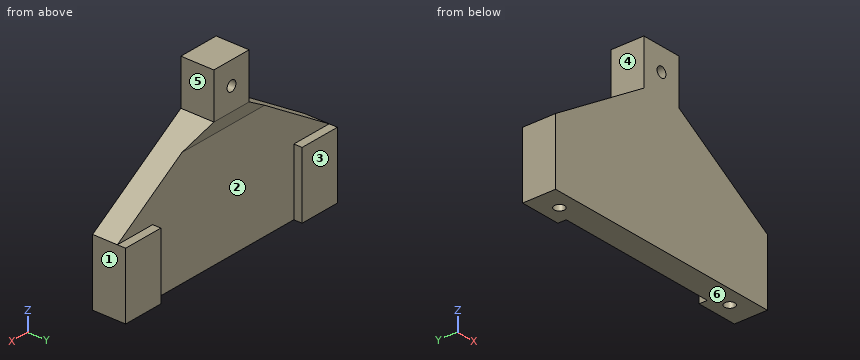
```python
from build123d import *

# Parameters (mm, degrees)
ESQUISSE1_W             = 60
ESQUISSE1_H             = 8
BOSS_EXTRU_1_DEPTH      = 60
ESQUISSE2_R             = 1.25
ENL_V_MAT_EXTRU_1_DEPTH = 15
ESQUISSE3_R             = 1.25
ENL_V_MAT_EXTRU_2_DEPTH = 15
ESQUISSE4_W             = 10
ESQUISSE4_H             = 11
ENL_V_MAT_EXTRU_3_DEPTH = 2
ENL_V_MAT_EXTRU_4_DEPTH = 52
CHANFREIN1_SIZE2        = 4.289013841
CHANFREIN1_SIZE         = 2


with BuildPart() as part:
    # Esquisse1 → Boss.-Extru.1 (new body)
    with BuildSketch(Plane.XY):
        with Locations((30, 4)):
            Rectangle(ESQUISSE1_W, ESQUISSE1_H)
    extrude(amount=BOSS_EXTRU_1_DEPTH)

    # Esquisse2 → Enlèv. mat.-Extru.1 (cut)
    with BuildSketch(Plane(origin=(0, 0, 0), x_dir=(-1, 0, 0), z_dir=(0, 0, -1))):
        with Locations((-54, 4)):
            Circle(ESQUISSE2_R)
        with Locations((-5.75, 4)):
            Circle(ESQUISSE2_R)
    extrude(amount=-ENL_V_MAT_EXTRU_1_DEPTH, mode=Mode.SUBTRACT)

    # Esquisse3 → Enlèv. mat.-Extru.2 (cut)
    with BuildSketch(Plane(origin=(0, 8, 0), x_dir=(1, 0, 0), z_dir=(0, 1, 0))):
        with Locations(Location((30, -37.5, 0), (0, 0, 270))):
            Circle(ESQUISSE3_R)
    extrude(amount=-ENL_V_MAT_EXTRU_2_DEPTH, mode=Mode.SUBTRACT)

    # Esquisse4 → Enlèv. mat.-Extru.3 (cut)
    with BuildSketch(Plane(origin=(0, 8, 0), x_dir=(1, 0, 0), z_dir=(0, 1, 0))):
        Polygon((0, -16), (10, -16), (10, 0), (50, 0), (50, -16), (60, -16), (60, -60), (0, -60), align=None)
        with Locations((30, -37.5)):
            Rectangle(ESQUISSE4_W, ESQUISSE4_H, mode=Mode.SUBTRACT)
    extrude(amount=-ENL_V_MAT_EXTRU_3_DEPTH, mode=Mode.SUBTRACT)

    # Esquisse5 → Enlèv. mat.-Extru.4 (cut)
    with BuildSketch(Plane(origin=(0, 6, 0), x_dir=(1, 0, 0), z_dir=(0, 1, 0))):
        Polygon((60, -16), (35, -32), (35, -43), (25, -43), (25, -32), (0, -16), (-21.594855386, -85.475485762), (75.414479662, -69.930764824), align=None)
    extrude(amount=-ENL_V_MAT_EXTRU_4_DEPTH, mode=Mode.SUBTRACT)

    # Chanfrein1
    chanfrein1_edges = [part.edges().sort_by_distance(p)[0] for p in [
        (30, 6, 32),
    ]]
    chanfrein1_side = [part.faces().sort_by_distance(p)[0] for p in [
        (30, 6.04, 32),
    ]]
    chamfer(chanfrein1_edges, length=CHANFREIN1_SIZE - 0.0001, length2=CHANFREIN1_SIZE2 - 0.0001, reference=chanfrein1_side[0])  # a hair under: the kernel refuses the full size


solid = part.part
```
Could you check a few things on this model? Use its own coordinates, in mm. Face numbers are marked on the shaded views. A direction names the side the tool comes from. Coordinates: 2 decimals unless noted, no trailing zeros. Write each loop counter-clockwise with the first axis right and the second up, starting at its lowest first coordinate (ties: lowest second). Pieces come first, ordered by that corner, then holes. Notation, with made-up numbers: (23, 59.5) -> (77, 59.5) arc R20 ccw to (77, 73.5) -> close; hole circle Ø4 at (78, 21.5). An arc over 180 degrees is marked (long way). Return JSON: item names as keys, results as strings.
(1) I need wall thicknesses on L1, parallel to Y at x = 54, z = 11; L2, parallel to X at y = 2.5, z = 39; L3, parallel to Y at x = 30, z = 9. Which ranges of each line are inside material? Lowest first, please.
Numbers:
{"L1": "y = 0 to 2.75, 5.25 to 8", "L2": "x = 25 to 35", "L3": "y = 0 to 6"}
(2) Which directions (+Z, -Z, +X, -X, +Y, -Y) give clear straight access to the entire face, cutting with the end or side of a thin tool? Please do the marked faces 4, 5 and 6.
Numbers:
{"face 4": "+Z, -X, +Y, -Y", "face 5": "+Z, +X, +Y, -Y", "face 6": "-Z, +X, -X, +Y, -Y"}
(3) I'm going to push flat-ended pins straight in: pin 1 (4 mm diameter, centred on y = 4, z = 36, fed in from +X); pin 2 (4 mm diameter, centred on y = 4.5, z = 31, fed in from -X); pin 3 (8.5 mm diameter, centred on x = 41.5, z = 18.5, fed in from +Y); pin 4 (3 mm diameter, centred on x = 54, y = 4, fed in from -Z). Where does each tip first touch, or does it pass through?
Numbers:
{"pin 1": "stops at x = 35", "pin 2": "stops at x = 20.31", "pin 3": "stops at y = 6", "pin 4": "stops at z = 0"}
(4) We'd pull the mould along X, two halves only. Please class the marked faces 1, 2 and 3: +X half, -X half, draft (parallel to the pull), parting line (faces both ways), or undercut.
Numbers:
{"face 1": "+X half", "face 2": "undercut", "face 3": "draft"}
(5) Imagine slicing it at B-B, the plane z = 37.5. Please give me the cut outline in (x, y), then the cut area to 3 significant figures.
Numbers:
{"outline": "(25, 0) -> (28.75, 0) -> (28.75, 8) -> (25, 8) -> close; (31.25, 0) -> (35, 0) -> (35, 8) -> (31.25, 8) -> close", "area": "60.0 mm2"}
(6) Imagine slicing it at D-D, the plane x = 54. Please give me the cut outline in (y, z), then the cut area to 3 significant figures.
Numbers:
{"outline": "(0, 0) -> (2.75, 0) -> (2.75, 15) -> (5.25, 15) -> (5.25, 0) -> (8, 0) -> (8, 16) -> (6, 16) -> (6, 19.84) -> (0, 19.84) -> close", "area": "114 mm2"}
(7) Imagine slicing it at C-C, the plane y = 1. Please give me the cut outline in (x, z), then the cut area to 3 significant figures.
Numbers:
{"outline": "(0, 0) -> (60, 0) -> (60, 16) -> (35, 32) -> (35, 43) -> (25, 43) -> (25, 32) -> (0, 16) -> close; hole circle Ø2.5 at (30, 37.5)", "area": "1,630 mm2"}
